Study the drawing (mm; zero at the part's minimum x, y, z) and answer. Give positions to 0.01 mm unless a question says otherwise; leave off trailing zeros. Order: outer loops, then holes, each group sorted by start corner. A loop starts at its lowest first (then second) coordinate and runs counter-clockwise, first axis right, second up. Notation, with made-up numbers: (86, 50) -> (129, 50) arc R22 cw to (129, 69) -> close; hole circle Ø7 at (-15.75, 3.25). An arc over 180 degrees is marked (long way). Answer as CSV lines item,"result". Start each with the question number.
1. Flat-ended cylindrical pins translate along their axes: pin 1 (2 mm diameter, centred on y = 8, z = 186, fed in from +X); pin 2 (21 mm diameter, centred on x = 2206.5, y = 35, fed in from +Z); pin 3 (5 mm diameter, centred on y = 15, z = 60.5, fed in from -X). Find the tip coordinate at first contact, or state that the pin passes through.
2. Find the intervals of material crossed by L1, parallel to X at y = 27.5, z = 269 (1 decimal); L2, parallel to X at y = 24, z = 291.5; L3, parallel to Z at x = 279, y = 65, in increasing order.
3. A cutting plane is placed at A-A (y = 54.5). Give the vertices of the cut face in (x, z) (1 decimal).
4. A cutting plane is placed at B-B (z = 243.5). Give the vertices of the cut face in (x, y) (1 decimal).
5. A cutting plane is placed at C-C (z = 337). Give the vertices of the cut face in (x, y), then the cut area to 3 significant figures.
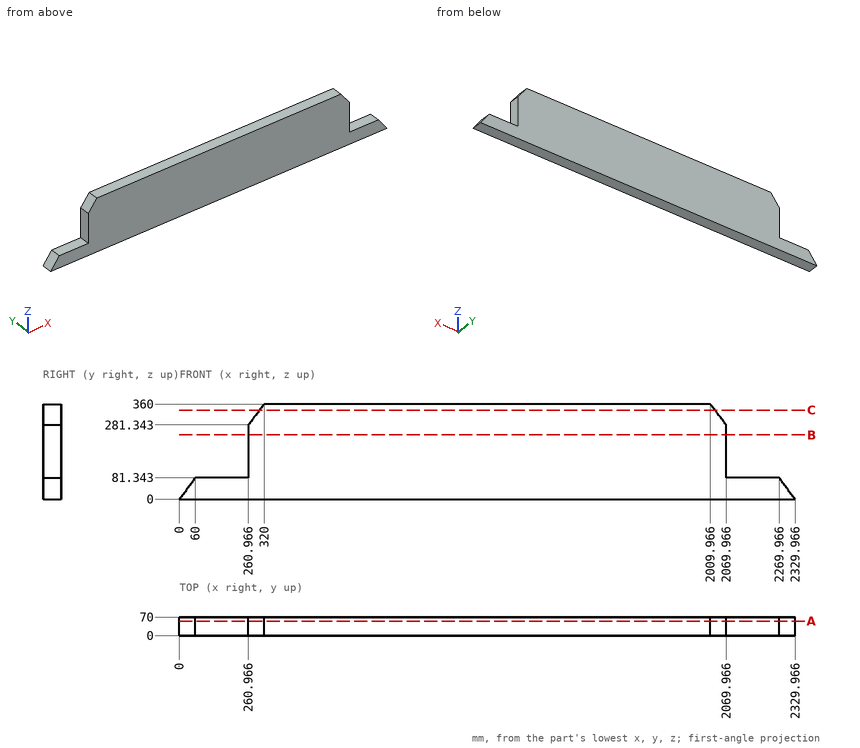
Answer sheet:
1,pin 1,"stops at x = 2069.97"
1,pin 2,"stops at z = 81.34"
1,pin 3,"stops at x = 42.78"
2,L1,"x = 261 to 2070"
2,L2,"x = 268.59 to 2062.22"
2,L3,"z = 0 to 305.37"
3,outline,"(0, 0) -> (2330, 0) -> (2270, 81.3) -> (2070, 81.3) -> (2070, 281.3) -> (2010, 360) -> (320, 360) -> (261, 281.3) -> (261, 81.3) -> (60, 81.3) -> close"
4,outline,"(261, 0) -> (2070, 0) -> (2070, 70) -> (261, 70) -> close"
5,outline,"(302.74, 0) -> (2027.51, 0) -> (2027.51, 70) -> (302.74, 70) -> close"
5,area,"121,000 mm^2"
